Can you work these out from the model? Positions are in its coordinate system, mm. A direction names the side the tool comes from. Give positions to 0.01 mm unless a question says otherwise; leave off trailing zeros. Loops run counter-clockwise (first coordinate to the right, second up) from the corner with the lowest first, then second, coordinate; pieces in that order, holes last. Notation, with made-up numbers: (3.25, 30) -> (16.25, 30) arc R12 ccw to (16.25, 42) -> close; hole circle Ø4 at (-36.75, 33.25). An arc over 180 degrees is marked (long way). Return JSON: item names as keys, results as strings. Group by question number.
Q1. Suppose I cut it at B-B, the plane z = 12. Please give me the cut outline in (x, y).
Q2. Suppose I cut it at C-C, the plane x = 53. Please give me the cut outline in (y, z), and give its area (3 significant figures).
Q3. Thinking about a two-plate mould opening in X: for faces 4 (the cylindrical face through (32.874, -22.788, 24.535)), 5 (the flat face through (4.2, 40.3, 27)), which applies, pulls with the +X half, pulls with the -X half, needs draft (parallel to the pull), parting line crosses it, or undercut?
Q4. I need wall thicknesses on line 1 along Y through (x, z) = (0, 3.8); line 2 along Z through (x, y) = (-7.5, 44.5); line 3 along X through (y, z) = (35, 24). Which ranges of each line are inside material? Lowest first, please. Write a range as [from, to].
Q5. Suppose I cut it at D-D, the plane y = -45. Please give me the cut outline in (x, z), and give its area (3 significant figures).
Q6. Suppose I cut it at A-A, the plane y = 48. Please give me the cut outline in (x, z).
Q7. Will these pins go through, and if not, where does the flat tip stop? pin 1 (1 mm diameter, centred on x = 7.5, z = 7, fed in from -Y); pin 2 (10 mm diameter, centred on x = -30.5, z = 10, fed in from +Y); pin 3 (12 mm diameter, centred on y = -36.5, z = 12, fed in from -X); pin 4 (1.5 mm diameter, centred on x = -10.5, y = 36, fed in from -Z).
Q8. Which directions (+Z, -Z, +X, -X, +Y, -Y) give clear straight access to the entire face, cutting with the end or side of a thin tool? Please do faces 1 (the cylindrical face through (-18.9, 46.29, 13.38)), 2 (the cylindrical face through (-37.37, 14.26, 24.54)), 3 (the cylindrical face through (29.1, -33, 24.5)).
```python
from build123d import *

# Parameters (mm, degrees)
SKETCH1_R            = 60
BOSS_EXTRUDE1_DEPTH  = 5
SKETCH2_R            = 60
SKETCH2_R_2          = 50
BOSS_EXTRUDE2_DEPTH  = 22
SKETCH3_R            = 60
SKETCH3_R_2          = 40
BOSS_EXTRUDE3_DEPTH  = 5
SKETCH4_R            = 12.5
CUT_EXTRUDE1_DEPTH   = 6
SKETCH5_R            = 4
CUT_EXTRUDE2_DEPTH   = 28
M6_CLEARANCE_HOLE1_D = 6.6


with BuildPart() as part:
    # Sketch1 → Boss-Extrude1 (new body)
    with BuildSketch(Plane.XY):
        Circle(SKETCH1_R)
    extrude(amount=BOSS_EXTRUDE1_DEPTH)

    # Sketch2 → Boss-Extrude2 (add)
    with BuildSketch(Plane.XY.offset(5)):
        Circle(SKETCH2_R)
        Circle(SKETCH2_R_2, mode=Mode.SUBTRACT)
    extrude(amount=BOSS_EXTRUDE2_DEPTH)

    # Sketch3 → Boss-Extrude3 (add)
    with BuildSketch(Plane.XY.offset(27)):
        Circle(SKETCH3_R)
        Circle(SKETCH3_R_2, mode=Mode.SUBTRACT)
    extrude(amount=-BOSS_EXTRUDE3_DEPTH)

    # Sketch4 → Cut-Extrude1 (cut, through all)
    with BuildSketch(Plane.XY.offset(5)):
        Circle(SKETCH4_R)
    extrude(amount=-CUT_EXTRUDE1_DEPTH, mode=Mode.SUBTRACT)

    # Sketch5 → Cut-Extrude2 (cut, through all)
    with BuildSketch(Plane.XY.offset(27)):
        with Locations((0, 40)):
            Circle(SKETCH5_R)
        with Locations((18.588926882, 35.418241026)):
            Circle(SKETCH5_R)
        with Locations((32.919354636, 22.722589869)):
            Circle(SKETCH5_R)
        with Locations((39.708354964, 4.82146721)):
            Circle(SKETCH5_R)
        with Locations((37.400649707, -14.184195482)):
            Circle(SKETCH5_R)
        with Locations((26.52490633, -29.940429927)):
            Circle(SKETCH5_R)
        with Locations((9.572626572, -38.837672697)):
            Circle(SKETCH5_R)
        with Locations((-9.572626572, -38.837672697)):
            Circle(SKETCH5_R)
        with Locations((-26.52490633, -29.940429927)):
            Circle(SKETCH5_R)
        with Locations((-37.400649707, -14.184195482)):
            Circle(SKETCH5_R)
        with Locations((-39.708354964, 4.82146721)):
            Circle(SKETCH5_R)
        with Locations((-32.919354636, 22.722589869)):
            Circle(SKETCH5_R)
        with Locations((-18.588926882, 35.418241026)):
            Circle(SKETCH5_R)
    extrude(amount=-CUT_EXTRUDE2_DEPTH, mode=Mode.SUBTRACT)

    # M6 Clearance Hole1 (through all)
    with Locations(Plane.XY.offset(27)):
        with Locations((0, 53), (37.476659403, 37.476659403), (53, 0), (37.476659403, -37.476659403), (0, -53), (-37.476659403, -37.476659403), (-53, 0), (-37.476659403, 37.476659403)):
            Hole(M6_CLEARANCE_HOLE1_D / 2)


solid = part.part
```
Ans:
{
 "1": {"outline": "circle Ø120 at (0, 0); hole (-49.98, -1.34) arc R50 ccw to (-36.29, -34.4) arc R3.3 ccw (long way) to (-34.4, -36.29) arc R50 ccw to (-1.34, -49.98) arc R3.3 ccw (long way) to (1.34, -49.98) arc R50 ccw to (34.4, -36.29) arc R3.3 ccw (long way) to (36.29, -34.4) arc R50 ccw to (49.98, -1.34) arc R3.3 ccw (long way) to (49.98, 1.34) arc R50 ccw to (36.29, 34.4) arc R3.3 ccw (long way) to (34.4, 36.29) arc R50 ccw to (1.34, 49.98) arc R3.3 ccw (long way) to (-1.34, 49.98) arc R50 ccw to (-34.4, 36.29) arc R3.3 ccw (long way) to (-36.29, 34.4) arc R50 ccw to (-49.98, 1.34) arc R3.3 ccw (long way) to start"},
 "2": {"outline": "(-28.12, 0) -> (-3.3, 0) -> (-3.3, 27) -> (-28.12, 27) -> close; (3.3, 0) -> (28.12, 0) -> (28.12, 27) -> (3.3, 27) -> close", "area": "1,340 mm^2"},
 "3": {"face 4": "undercut", "face 5": "needs draft"},
 "4": {"line 1": "y = [-60, -56.3], [-49.7, -12.5], [12.5, 36], [44, 49.7], [56.3, 60]", "line 2": "z = [0, 5], [22, 27]", "line 3": "x = [-48.73, -39.66], [-35.3, -22.57], [22.57, 35.3], [39.66, 48.73]"},
 "5": {"outline": "(-39.69, 0) -> (39.69, 0) -> (39.69, 27) -> (-39.69, 27) -> close; hole (-21.79, 5) -> (21.79, 5) -> (21.79, 22) -> (-21.79, 22) -> close", "area": "1,400 mm^2"},
 "6": {"outline": "(-36, 0) -> (36, 0) -> (36, 27) -> (-36, 27) -> close; hole (-14, 5) -> (14, 5) -> (14, 22) -> (-14, 22) -> close"},
 "7": {"pin 1": "stops at y = -59.59", "pin 2": "stops at y = 54.31", "pin 3": "stops at x = -51.67", "pin 4": "stops at z = 0"},
 "8": {"face 1": "none", "face 2": "+Z", "face 3": "+Z, -Z"}
}
